Geometry: see drawing. Coordinates: mm, zero at the bounding-box minimum. A direction names the side the tool comes from. Coordinates: 2 decimals unless noted, no trailing zeros. Write each loop counter-clockwise with the first axis right and the second up, starting at its lowest first coordinate (ties: lowest second). Pieces come first, ordered by that corner, then holes. Notation, with made-up numbers: (-37.5, 19.25) -> (-15.5, 19.25) arc R22 ccw to (-15.5, 26.25) -> close; hole circle Ø1 at (75.25, 30). An arc over 180 degrees is marked (long way). Use one line per item in the form item = value. Start each with the question number.
(1) Cut plane B-B on x = 0.7. Return the cut outline in (y, z).
(2) Cut plane C-C on y = 1.25. Return the cut outline in (x, z).
(3) Ray query, line 1 along Y through (x, z) = (2, 0.75); line 2 along Y through (x, z) = (1.35, 1.8) (1 decimal); line 3 along X through (y, z) = (5, 1.85). Return the intervals inside material, ascending.
(4) Set-up query: the marked faces 1, 2, 3, 4 and 5. Return all of +Z, -Z, +X, -X, +Y, -Y with unobstructed straight access to the full face (end or side cutting, diameter ignored); none if empty.
(5) Cut plane D-D on z = 1.8. Return the cut outline in (x, y).
(6) Pull-direction query (X, two-part tool) for the marked faces 6, 7 and 8; classes: released by +X, released by -X, zero draft, split by the parting line, or undercut.
(7) Cut plane A-A on z = 2.55. Return the cut outline in (x, y), plus the area to 3 significant figures.
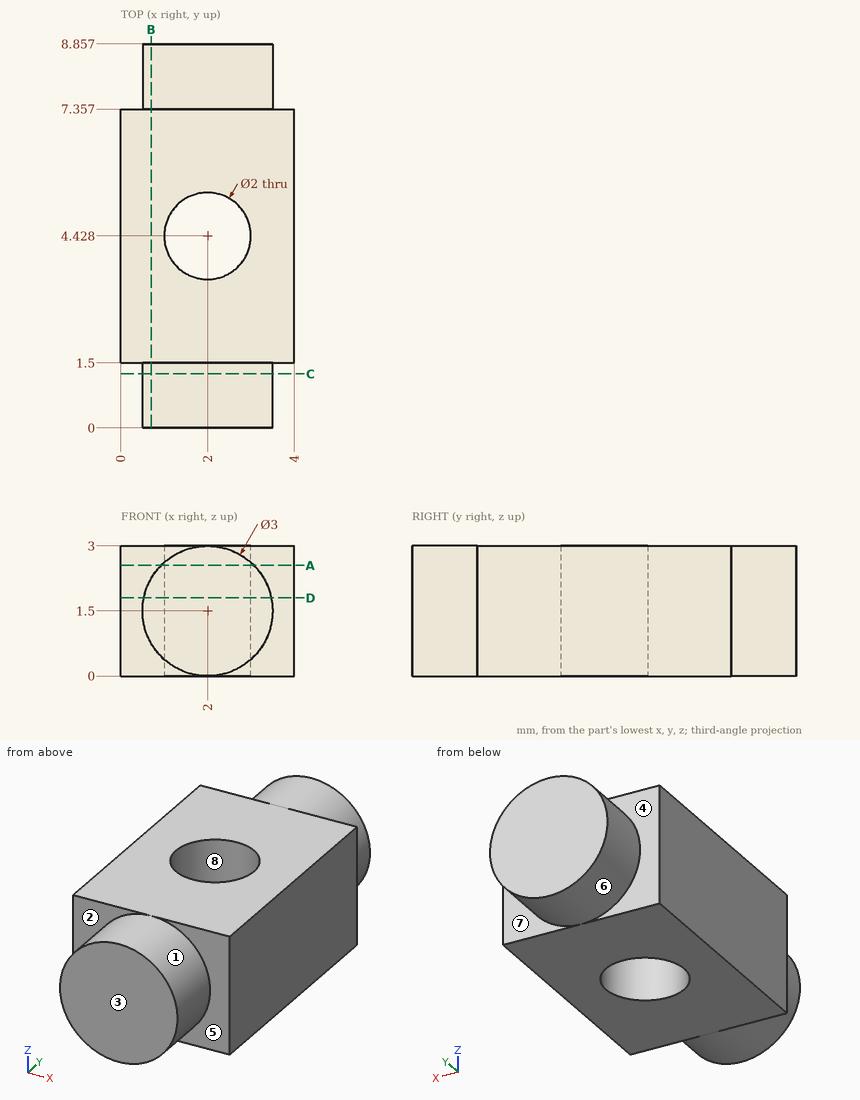
Values:
q1.outline = (0, 0.75) -> (1.5, 0.75) -> (1.5, 0) -> (7.36, 0) -> (7.36, 0.75) -> (8.86, 0.75) -> (8.86, 2.25) -> (7.36, 2.25) -> (7.36, 3) -> (1.5, 3) -> (1.5, 2.25) -> (0, 2.25) -> close
q2.outline = circle Ø3 at (2, 1.5)
q3.line_1 = 0 to 3.43, 5.43 to 8.86
q3.line_2 = 0 to 3.7, 5.2 to 8.9
q3.line_3 = 0 to 1.18, 2.82 to 4
q4.face_1 = -Y
q4.face_2 = -X, -Y
q4.face_3 = +Z, -Z, +X, -X, -Y
q4.face_4 = -X, +Y
q4.face_5 = +X, -Y
q5.outline = (0, 1.5) -> (0.53, 1.5) -> (0.53, 0) -> (3.47, 0) -> (3.47, 1.5) -> (4, 1.5) -> (4, 7.36) -> (3.47, 7.36) -> (3.47, 8.86) -> (0.53, 8.86) -> (0.53, 7.36) -> (0, 7.36) -> close; hole circle Ø2 at (2, 4.43)
q6.face_6 = split by the parting line
q6.face_7 = zero draft
q6.face_8 = undercut
q7.outline = (0, 1.5) -> (0.93, 1.5) -> (0.93, 0) -> (3.07, 0) -> (3.07, 1.5) -> (4, 1.5) -> (4, 7.36) -> (3.07, 7.36) -> (3.07, 8.86) -> (0.93, 8.86) -> (0.93, 7.36) -> (0, 7.36) -> close; hole circle Ø2 at (2, 4.43)
q7.area = 26.7 mm2
